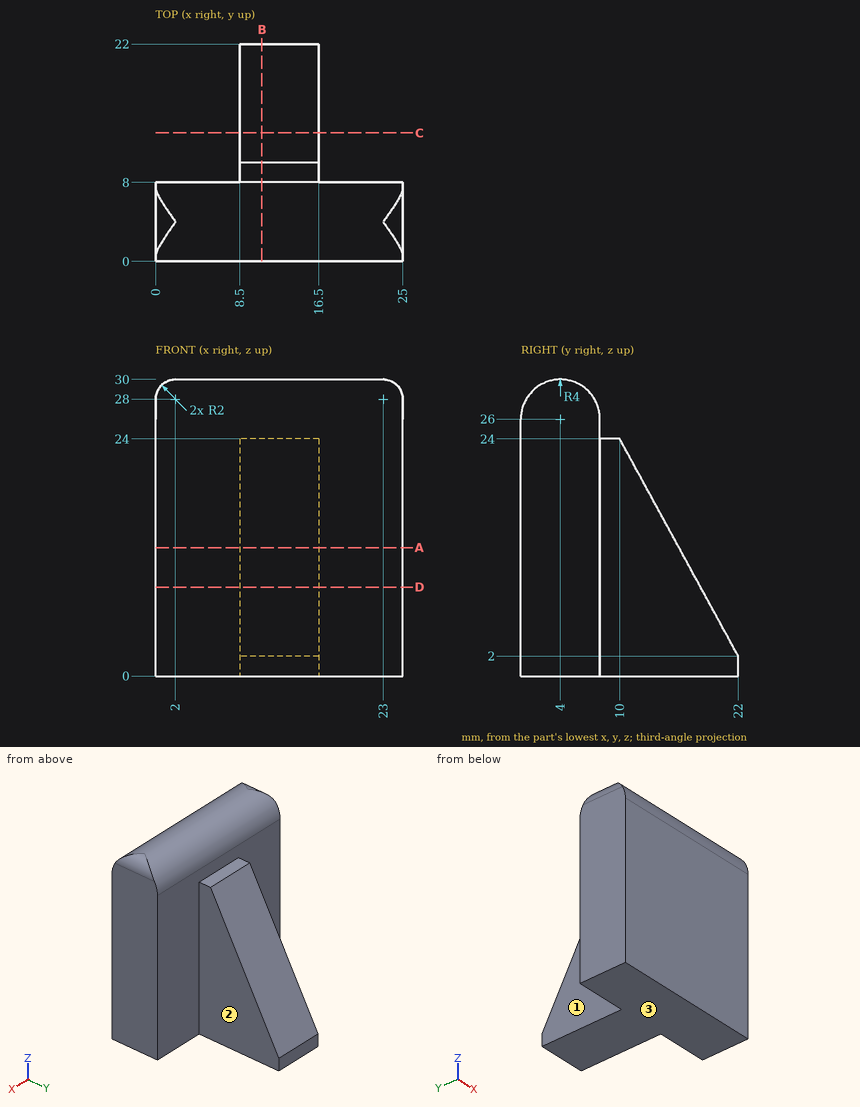
Geometry check sheet. Reference: drawing and pictorial views, mm from the part's lowest x, y, z. A direction names the side the tool comes from. Give positions to 0.01 mm unless a question says otherwise; leave off trailing zeros. Loops run counter-clockwise (first coordinate to the right, second up) from the corner with the lowest first, then second, coordinate; pieces in that order, holes last. Notation, with made-up numbers: (42.25, 61.5) - (75.25, 61.5) arc R13 cw to (75.25, 76.5) - close; hole circle Ø3 at (61, 11). An arc over 180 degrees is marked (long way). One line per question, with ' | ' between items. Start each with the question number.
1. Cross-section at D-D, the plane z = 9. Enter the section's corners in (x, y).
2. Cross-section at C-C, the plane y = 13. Enter the section's corners in (x, z).
3. Set-up check for the marked faces 1, 2 and 3: record each of +Z, -Z, +X, -X, +Y, -Y from which the full face is reachable in a straight line by a thin tool's end or side.
4. Cross-section at A-A, the plane z = 13. Enter the section's corners in (x, y).
5. Gauge pin test, flat ends, axial feed: pin 1 Ø12 at (x, z) = (16.5, 3.5) entering from +Y; pin 2 Ø2 at (x, y) = (10.5, 18) entering from +Z; pin 3 Ø4 at (x, z) = (15, 5) entering from +Y; pin 4 Ø4 at (y, z) = (11.5, 12) entering from +X. Record the tip position at first contact, or that the pin passes through.
6. Material ranges on line 1 along Y through (x, z) = (1.5, 20.5); line 2 along X through (y, z) = (10, 9.5); line 3 along Z through (x, y) = (16.25, 9.75), recorded low to high. Write a range as [from, to].
7. Cross-section at B-B, the plane x = 10.75. Enter the section's corners in (y, z).
Check result:
1) outline: (0, 0) - (25, 0) - (25, 8) - (16.5, 8) - (16.5, 18.18) - (8.5, 18.18) - (8.5, 8) - (0, 8) - close
2) outline: (8.5, 0) - (16.5, 0) - (16.5, 18.5) - (8.5, 18.5) - close
3) face 1: +Z, -Z, -X, +Y | face 2: +Z, -Z, +X, +Y | face 3: -Z, +X, -X, +Y, -Y
4) outline: (0, 0) - (25, 0) - (25, 8) - (16.5, 8) - (16.5, 16) - (8.5, 16) - (8.5, 8) - (0, 8) - close
5) pin 1: stops at y = 22 | pin 2: stops at z = 11.17 | pin 3: stops at y = 21.45 | pin 4: stops at x = 16.5
6) line 1: y = [0, 8] | line 2: x = [8.5, 16.5] | line 3: z = [0, 24]
7) outline: (0, 0) - (22, 0) - (22, 2) - (10, 24) - (8, 24) - (8, 26) arc R4 ccw to (0, 26) - close
